Check sheet for the modelled part. Datum: model origin and axes. Units: mm. Round coordinates to 2 decimals unless told otherwise and drop trailing zeros. Loops run counter-clockwise (first coordinate to the right, second up) from the corner with the lowest first, then second, coordinate; pieces in that order, holes last. Notation, with made-up numbers: (50, 37.25) -> (94, 37.25) arc R28 cw to (94, 72.25) -> close; hole circle Ø3 at (13.25, 66.5). An arc over 180 degrees is marked (long way). One line per question, with ' | ' between items.
```python
from build123d import *

# Parameters (mm, degrees)
F0_W     = 5
F0_H     = 20
F1_DEPTH = 100
F2_R     = 2
F3_DEPTH = 25
F4_R     = 2.5
F5_DEPTH = 5.001


with BuildPart() as f1:
    # F0 (on Front) → F1 (new body)
    with BuildSketch(Plane.XZ):
        with Locations((2.5, -10)):
            Rectangle(F0_W, F0_H)
    extrude(amount=F1_DEPTH)

    # F2 (on face) → F3 (cut)
    with BuildSketch(Plane(origin=(0, 0, 0), x_dir=(-1, 0, 0), z_dir=(0, 1, 0))):
        with Locations((-2.5, -10)):
            Circle(F2_R)
    extrude(amount=-F3_DEPTH, mode=Mode.SUBTRACT)

    # F4 (on face) → F5 (cut, through all)
    with BuildSketch(Plane.YZ.offset(5)):
        with Locations((-84.955528, -10)):
            Circle(F4_R)
    extrude(amount=-F5_DEPTH, mode=Mode.SUBTRACT)


solid = f1.part
```
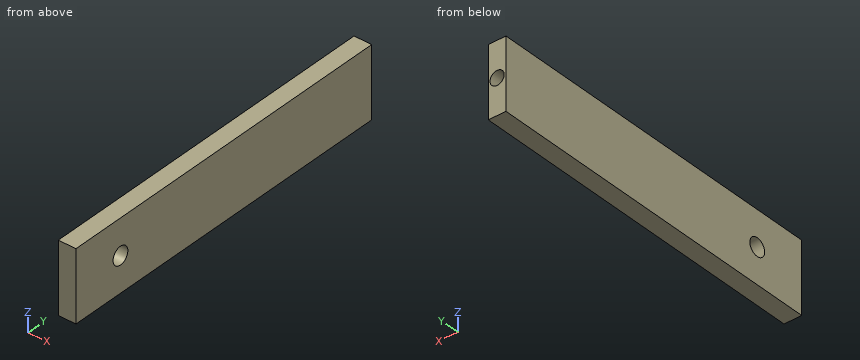
(1) Sectioned sample at A-A, the plane x = 2.5. Record the cut outline in (y, z).
Answer:
outline: (-100, -20) -> (0, -20) -> (0, -12) -> (-25, -12) -> (-25, -8) -> (0, -8) -> (0, 0) -> (-100, 0) -> close; hole circle Ø5 at (-84.96, -10)
(2) Scan lines: probe 1 along Z at (x, y) = (2.5, -13.25); probe 2 along Z at (x, y) = (3.8, -13.5); probe 3 along Y at (x, z) = (3.55, -10.5). Record each from-to range of solid material in increasing order.
Answer:
probe 1: z = -20 to -12, -8 to 0 | probe 2: z = -20 to -11.52, -8.48 to 0 | probe 3: y = -100 to -87.41, -82.51 to -25
(3) Sectioned sample at C-C, the plane y = -12. Record the cut outline in (x, z), and give its area (3 significant figures).
Answer:
outline: (0, -20) -> (5, -20) -> (5, 0) -> (0, 0) -> close; hole circle Ø4 at (2.5, -10) | area: 87.4 mm2
(4) Go/stop test with a flat-tipped pin: pin 1 (4.5 mm diameter, centred on y = -84.96, z = -10, fed in from -X). Record where the tip stops, or that it passes through.
Answer:
pin 1: passes through
(5) Sectioned sample at B-B, the plane z = -10. Record the cut outline in (x, y).
Answer:
outline: (0, -100) -> (5, -100) -> (5, -87.46) -> (0, -87.46) -> close; (0, -82.46) -> (5, -82.46) -> (5, 0) -> (4.5, 0) -> (4.5, -25) -> (0.5, -25) -> (0.5, 0) -> (0, 0) -> close
